```python
from build123d import *

# Parameters (mm, degrees)
SKETCH1_R           = 20
BOSS_EXTRUDE4_DEPTH = 20
SKETCH1_10_R        = 10
SKETCH1_10_R_2      = 7.5
BOSS_EXTRUDE5_DEPTH = 20
SKETCH1_11_R        = 15
CUT_EXTRUDE1_DEPTH  = 20
BOSS_EXTRUDE6_DEPTH = 12
BOSS_EXTRUDE7_DEPTH = 3
FILLET1_R           = 1.5


with BuildPart() as part:
    # Sketch1 → Boss-Extrude4 (new body)
    with BuildSketch(Plane.XY):
        Circle(SKETCH1_R)
    extrude(amount=BOSS_EXTRUDE4_DEPTH)

    # Sketch1_11 → Cut-Extrude1 (cut)
    with BuildSketch(Plane.XY):
        Circle(SKETCH1_11_R)
    extrude(amount=CUT_EXTRUDE1_DEPTH, mode=Mode.SUBTRACT)



with BuildPart() as body_2:
    # Sketch1_10 → Boss-Extrude5 (new body)
    with BuildSketch(Plane.XY):
        with Locations((-70, 0)):
            Circle(SKETCH1_10_R)
        with Locations((-70, 0)):
            Circle(SKETCH1_10_R_2, mode=Mode.SUBTRACT)
        with Locations((22, -36)):
            Circle(SKETCH1_10_R)
        with Locations((22, -36)):
            Circle(SKETCH1_10_R_2, mode=Mode.SUBTRACT)
    extrude(amount=BOSS_EXTRUDE5_DEPTH)


with BuildPart() as part_1:
    add(part.part)

    add(body_2.part)  # Boss-Extrude6 merges body 2
    # Sketch1_12 → Boss-Extrude6 (add)
    with BuildSketch(Plane.XY):
        with BuildLine():
            ThreePointArc((-67.619047619, 9.712418121), (-64.207085766, 8.151205106), (-61.610700763, 5.442394539))
            ThreePointArc((-61.610700763, 5.442394539), (-38.89416694, 4.977846482), (-16.902840155, 10.690836951))
            ThreePointArc((-16.902840155, 10.690836951), (-13.734956085, 14.537915303), (-9.714285714, 17.482352618))
            ThreePointArc((-9.714285714, 17.482352618), (-37.932007586, 8.122402385), (-67.619047619, 9.712418121))
        make_face()
        with BuildLine():
            ThreePointArc((-14.595467543, -13.673782476), (-37.607048321, -6.216745586), (-61.791440547, -5.711352878))
            ThreePointArc((-61.791440547, -5.711352878), (-64.474228629, -8.334617613), (-67.934982867, -9.784462389))
            ThreePointArc((-67.934982867, -9.784462389), (-22.262897918, -13.560739124), (13.842794911, -41.784462389))
            ThreePointArc((13.842794911, -41.784462389), (12.285119236, -38.370884169), (12.095188973, -34.623512255))
            ThreePointArc((12.095188973, -34.623512255), (4.201963756, -26.450336843), (-4.733552286, -19.431764787))
            ThreePointArc((-4.733552286, -19.431764787), (-10.084212511, -17.271614228), (-14.595467543, -13.673782476))
        make_face()
        with BuildLine():
            ThreePointArc((30.614150003, -30.920982406), (23.463789692, -15.074619609), (19.905470006, 1.94223167))
            ThreePointArc((19.905470006, 1.94223167), (19.976353522, 0.972265368), (20, 0))
            ThreePointArc((20, 0), (19.596577822, -3.996765901), (18.402586233, -7.832293401))
            ThreePointArc((18.402586233, -7.832293401), (21.047204692, -17.304888513), (24.793712928, -26.398168504))
            ThreePointArc((24.793712928, -26.398168504), (28.135861436, -28.103722115), (30.614150003, -30.920982406))
        make_face()
    extrude(amount=BOSS_EXTRUDE6_DEPTH)

    # Sketch1_13 → Boss-Extrude7 (add)
    with BuildSketch(Plane.XY):
        with BuildLine():
            ThreePointArc((-61.610700763, 5.442394539), (-60.411126438, 2.837869591), (-60, 0))
            ThreePointArc((-60, 0), (-60.458365063, -2.992858622), (-61.791440547, -5.711352878))
            ThreePointArc((-61.791440547, -5.711352878), (-37.607048321, -6.216745586), (-14.595467543, -13.673782476))
            ThreePointArc((-14.595467543, -13.673782476), (-19.910914517, -1.885598869), (-16.902840155, 10.690836951))
            ThreePointArc((-16.902840155, 10.690836951), (-38.89416694, 4.977846482), (-61.610700763, 5.442394539))
        make_face()
        with BuildLine():
            ThreePointArc((18.402586233, -7.832293401), (8.963679846, -17.878826685), (-4.733552286, -19.431764787))
            ThreePointArc((-4.733552286, -19.431764787), (4.201963756, -26.450336843), (12.095188973, -34.623512255))
            ThreePointArc((12.095188973, -34.623512255), (16.563457073, -27.606907543), (24.793712928, -26.398168504))
            ThreePointArc((24.793712928, -26.398168504), (21.047204692, -17.304888513), (18.402586233, -7.832293401))
        make_face()
    extrude(amount=BOSS_EXTRUDE7_DEPTH)

    # Fillet1
    fillet1_edges = [part_1.edges().sort_by_distance(p)[0] for p in [
        (-61.610700763, 5.442394539, 7.5),
        (-16.902840155, 10.690836951, 7.5),
        (-4.733552286, -19.431764787, 7.5),
        (-14.595467543, -13.673782476, 7.5),
        (-61.791440547, -5.711352878, 7.5),
        (12.095188973, -34.623512255, 7.5),
        (18.402586233, -7.832293401, 7.5),
        (24.793712928, -26.398168504, 7.5),
    ]]
    fillet(fillet1_edges, radius=FILLET1_R)


solid = part_1.part
```
For this review, take the finished solid that the model builds, in its own axes (mm). A direction names the side the tool comes from. Round coordinates to 2 decimals unless told otherwise and drop trailing zeros. Write each loop counter-clockwise with the first axis right and the second up, starting at its lowest first coordinate (ties: lowest second). Pieces come first, ordered by that corner, then holes. Notation, with made-up numbers: M -15,17 L 1,17 A32 ccw 1,54 Z; hole C -26.5,29.5 d5. An arc over 180 degrees is marked long. One line per item, written item: value. Start each with the question number.
(1) The part is to be moulded in two halves that separate along X. For faces 1 (the flat face through (26, -29, 20)), 2 (the cylindrical face through (21.2, -17.74, 7.44)), 3 (the cylindrical face through (-77.493, 0.33, 9.86)), say which applies: released by +X, released by -X, zero draft, split by the parting line, or undercut.
(2) We need section B-B (z = 17). Give the boundary of the cut face in (x, y), and give its area (3 significant figures).
(3) Insertion check: pin 1 (8 mm diameter, centred on y = -14, z = 7.5, fed in from +X); pin 2 (3 mm diameter, centred on y = 3, z = 7.5, fed in from -X); pin 3 (24 mm diameter, centred on x = 22, y = -36, fed in from +Z); pin 4 (10 mm diameter, centred on x = -3, z = 7.5, fed in from -Y). Each pin has a flat end and moves straight along its axis. Give the tip position at first contact, or say it passes through.
(4) Machinability: for faces 4 (the flat face through (23, -16, 12)), 5 (the cylindrical face through (-80, 0, 12)), 6 (the flat face through (-38.8, 7.7, 12)), 7 (the cylindrical face through (-14.985, 0.66, 9.86)), which of the approach directions +Z, -Z, +X, -X, +Y, -Y give a long, thin tool a straight path to every point of the face, cutting with its end or side? Answer none if there is none.
(5) We need section C-C (y = 0). Give the boundary of the cut face in (x, z).
(6) We need section D-D (y = -36). Give the boundary of the cut face in (x, z).
(7) Wall thickness on line 1 (X direction, y = -0.5, z = 16.25); line 2 (Y direction, x = 0, z = 4.5); line 3 (Y direction, x = -70, z = 15): over which ranges is each line inside the solid? List them lowest first.
(8) We need section A-A (x = -70). Give the boundary of the cut face in (y, z).
Result:
1. face 1: zero draft
1. face 2: undercut
1. face 3: undercut
2. outline: C -70,0 d20; C 0,0 d40; C 22,-36 d20; hole C -70,0 d15; hole C 0,0 d30; hole C 22,-36 d15
2. area: 825 mm²
3. pin 1: x = 24.48
3. pin 2: x = -79.89
3. pin 3: z = 20
3. pin 4: y = -28.5
4. face 4: +Z, +X
4. face 5: +Z
4. face 6: +Z, +Y
4. face 7: +Z, -Z
5. outline: M -80,0 L -77.5,0 L -77.5,20 L -80,20 Z; M -62.5,0 L -15,0 L -15,20 L -20,20 L -20,3 L -60,3 L -60,20 L -62.5,20 Z; M 15,0 L 20.12,0 L 20.12,12 L 20,12 L 20,20 L 15,20 Z
6. outline: M 9.33,0 L 14.5,0 L 14.5,20 L 12,20 L 12,12 L 9.33,12 Z; M 29.5,0 L 32,0 L 32,20 L 29.5,20 Z
7. line 1: -79.99 to -77.48, -62.52 to -60.01, -19.99 to -14.99, 14.99 to 19.99
7. line 2: -26.77 to -22.9, -20.13 to -15, 15 to 20
7. line 3: -10 to -7.5, 7.5 to 10
8. outline: M -10,0 L -7.5,0 L -7.5,20 L -10,20 Z; M 7.5,0 L 10,0 L 10,20 L 7.5,20 Z
